Source: CAD feature listing. Evaluate the final solid. Frame: model axes, mm. Round coordinates to 2 decimals unless told otherwise and drop trailing zeros. Order: outer loops, then holes, each group sorted by start corner. A loop starts at its lowest first (then second) coordinate and runs counter-clockwise, first axis right, second up. Notation, with made-up numbers: (1.5, 23) -> (39.5, 23) arc R18 cw to (39.5, 38) -> close; hole circle Ø6 at (35, 22). An arc over 180 degrees is marked (long way). Write item = value, one per line. Start each with the question number.
(1) Draft query along Y for faces 1 (the face through (-57.521, -44.105, 7.196)), 2 (the face through (40.136, -77.167, -13.35)), 3 (the face through (-33, 65, 29.245)). Return one class per face: released by +Y, released by -Y, zero draft, split by the parting line, or undercut.
(2) Cut plane C-C on z = 24. Return the cut outline in (x, y), then the cut area to 3 significant figures.
(3) Cut plane D-D on z = 0. Return the cut outline in (x, y).
(4) Contact query for flat-ended pins moving along their axis: pin 1 Ø12 at (x, z) = (-22, 4.5) entering from -Y; pin 2 Ø10 at (y, z) = (-64.5, 6.5) entering from -X; pin 3 Ø8 at (x, z) = (63, 3.5) entering from -Y. Output: stop coordinate, or through.
(5) Ray query, line 1 (Y direction, x = 0, z = 2.5); line 2 (Y direction, x = -32, z = 0); line 3 (X direction, y = 8.5, z = 13). Return the intervals inside material, ascending.
(6) Cut plane A-A on x = 0. Return the cut outline in (y, z).
from build123d import *

# Parameters (mm, degrees)
SKETCH1_R           = 30
SKETCH1_R_2         = 25
BOSS_EXTRUDE1_DEPTH = 15
SKETCH2_R           = 7.5
SCALE1_SCALE        = 1.9329
SCALE2_SCALE        = 1.5


with BuildPart() as part:
    # Sketch1 → Boss-Extrude1 (new body)
    with BuildSketch(Plane.XY):
        Circle(SKETCH1_R)
        Circle(SKETCH1_R_2, mode=Mode.SUBTRACT)
    extrude(amount=BOSS_EXTRUDE1_DEPTH)

    # Sketch2 → Cut-Revolve1 (revolve, cut)
    with BuildSketch(Plane(origin=(0, 0, 0), x_dir=(0, 0, -1), z_dir=(1, 0, 0)), mode=Mode.PRIVATE) as cut_revolve1_sk:
        with Locations((-7.5, 33)):
            Circle(SKETCH2_R)
    revolve(cut_revolve1_sk.sketch.rotate(Axis((0, 0, 25.257665056), (0, 0, -1)), 90), axis=Axis((0, 0, 25.257665056), (0, 0, -1)), mode=Mode.SUBTRACT)


with BuildPart() as part_1:
    # Scale1: scaled about (0, 0, 7.5)
    add(part.part.scale(SCALE1_SCALE).moved(Location((0, 0, -6.99675))))


with BuildPart() as part_2:
    # Scale2: scaled about (0, 0, 7.5)
    add(part_1.part.scale(SCALE2_SCALE).moved(Location((0, 0, -3.75))))


solid = part_2.part
Evaluation:
q1.face_1 = undercut
q1.face_2 = split by the parting line
q1.face_3 = zero draft
q2.outline = circle Ø163.03 at (0, 0); hole circle Ø144.97 at (0, 0)
q2.area = 4,370 mm^2
q3.outline = circle Ø150.54 at (0, 0); hole circle Ø144.97 at (0, 0)
q4.pin_1 = -73.11
q4.pin_2 = -43.94
q4.pin_3 = -45.35
q5.line_1 = -74.52 to -72.48, 72.48 to 74.52
q5.line_2 = -68.13 to -65.04, 65.04 to 68.13
q5.line_3 = -74.15 to -71.98, 71.98 to 74.15
q6.outline = (-86.98, -14.25) -> (-72.48, -14.25) -> (-72.48, 29.25) -> (-86.98, 29.25) -> (-86.98, 27.43) arc R21.75 cw to (-86.98, -12.43) -> close; (72.48, -14.25) -> (86.98, -14.25) -> (86.98, -12.43) arc R21.75 cw to (86.98, 27.43) -> (86.98, 29.25) -> (72.48, 29.25) -> close
